Geometry: see drawing. Coordinates: mm, zero at the bounding-box minimum. A direction names the side the tool comes from. Give positions to 0.01 mm unless a question says otherwise; leave off trailing zeros. Write each loop counter-clockwise with the first axis right and the second up, starting at its lowest first coordinate (ties: lowest second). Pieces come first, ordered by that corner, then holes. Notation, with made-up numbers: (-14, 84) - (44, 84) arc R24 ccw to (44, 95) - close; hole circle Ø11 at (-18, 60). An arc over 180 degrees is marked (long way). Use CSV: the item, a comma, the result in double quotes. Start each with the question number.
(1) Draft query along X for the marked faces 1, 2 and 3. Return one class per face: released by +X, released by -X, zero draft, split by the parting line, or undercut.
(2) First-contact query: pin 1 Ø4.5 at (x, z) = (3, 8) entering from +Y. Flat tip, straight axial feed; report the tip coordinate or a pass-through.
(3) Section B-B on z = 14. Output: boundary loops of the cut face in (x, y), and give its area (3 significant figures).
(4) Reachability of the marked faces 4, 5 and 6 from +Z, -Z, +X, -X, +Y, -Y: full face, straight path, thin tool, end or side. Return the list, or none.
(5) Section D-D on z = 9.5. Output: boundary loops of the cut face in (x, y).
(6) Line query: probe 1 along Z at (x, y) = (3.2, 0.7); probe 2 along X at (y, z) = (1.15, 15.5) (1 decimal); probe 3 along X at (y, z) = (0.75, 14). Output: solid intervals per line, ascending. Write a range as [from, to].
(7) Section A-A on x = 16.8. Output: boundary loops of the cut face in (y, z).
(8) Section C-C on y = 0.3. Output: boundary loops of the cut face in (x, z), and give its area (3 significant figures).
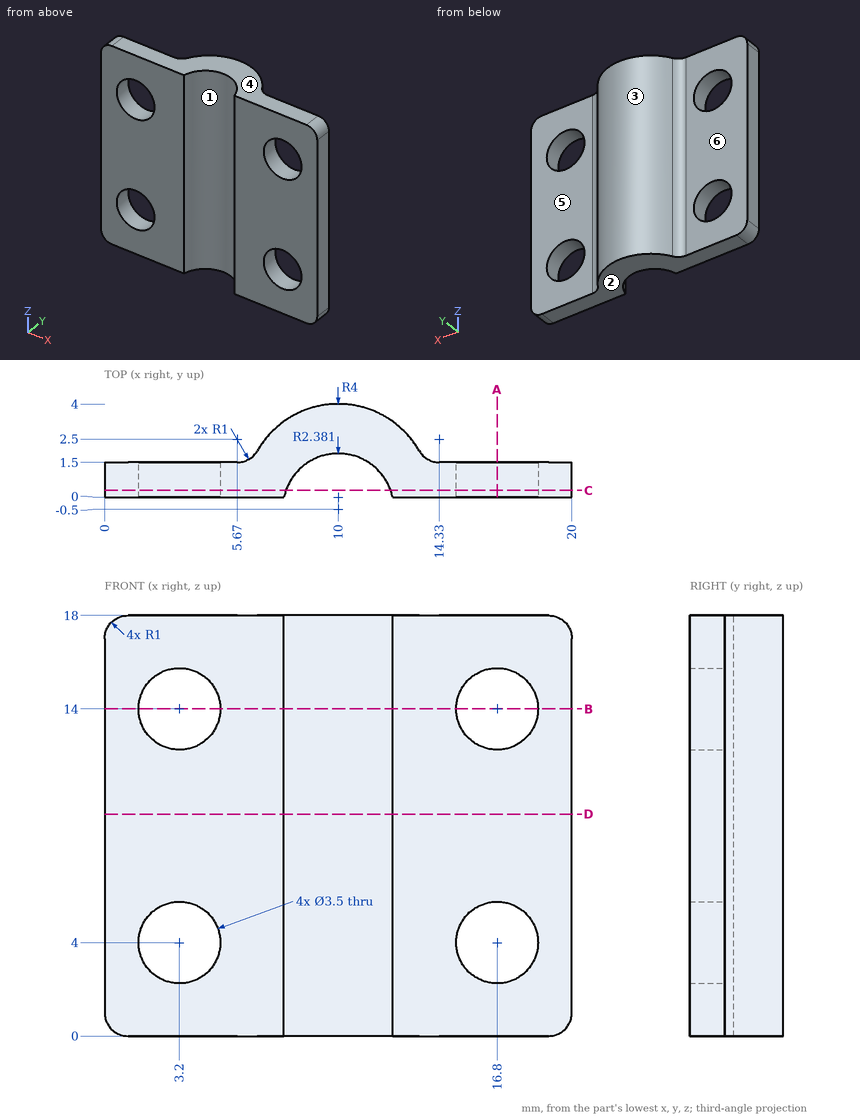
Check values:
1,face 1,"undercut"
1,face 2,"zero draft"
1,face 3,"split by the parting line"
2,pin 1,"stops at y = 1.5"
3,outline,"(0, 0) - (1.45, 0) - (1.45, 1.5) - (0, 1.5) - close; (4.95, 0) - (7.67, 0) arc R2.38 cw to (12.33, 0) - (15.05, 0) - (15.05, 1.5) - (14.33, 1.5) arc R1 cw to (13.46, 2) arc R4 ccw to (6.54, 2) arc R1 cw to (5.67, 1.5) - (4.95, 1.5) - close; (18.55, 0) - (20, 0) - (20, 1.5) - (18.55, 1.5) - close"
3,area,"26.5 mm²"
4,face 4,"+Z, +X, -X, +Y, -Y"
4,face 5,"+Z, -Z, +X, +Y"
4,face 6,"+Z, -Z, -X, +Y"
5,outline,"(0, 0) - (7.67, 0) arc R2.38 cw to (12.33, 0) - (20, 0) - (20, 1.5) - (14.33, 1.5) arc R1 cw to (13.46, 2) arc R4 ccw to (6.54, 2) arc R1 cw to (5.67, 1.5) - (0, 1.5) - close"
6,probe 1,"z = [0, 2.25], [5.75, 12.25], [15.75, 18]"
6,probe 2,"x = [0, 2.3], [4.1, 8.3], [11.7, 15.9], [17.7, 20]"
6,probe 3,"x = [0, 1.45], [4.95, 7.97], [12.03, 15.05], [18.55, 20]"
7,outline,"(0, 0) - (1.5, 0) - (1.5, 2.25) - (0, 2.25) - close; (0, 5.75) - (1.5, 5.75) - (1.5, 12.25) - (0, 12.25) - close; (0, 15.75) - (1.5, 15.75) - (1.5, 18) - (0, 18) - close"
8,outline,"(0, 1) arc R1 ccw to (1, 0) - (7.76, 0) - (7.76, 18) - (1, 18) arc R1 ccw to (0, 17) - close; (12.24, 0) - (19, 0) arc R1 ccw to (20, 1) - (20, 17) arc R1 ccw to (19, 18) - (12.24, 18) - close; hole circle Ø3.5 at (3.2, 4); hole circle Ø3.5 at (3.2, 14); hole circle Ø3.5 at (16.8, 4); hole circle Ø3.5 at (16.8, 14)"
8,area,"240 mm²"
